Can you work these out from the model? Positions are in its coordinate system, mm. A direction names the side the tool comes from. Give positions to 0.01 mm unless a question says otherwise; leave off trailing zeros. Order: outer loops, then holes, each group sorted by start corner. A loop starts at its lowest first (then second) coordinate and runs counter-clockwise, first axis right, second up. Notation, with made-up numbers: (-19, -1.5) -> (-12, -1.5) arc R29 ccw to (-12, 35.5) -> close; hole circle Ø1 at (-1.75, 15). An arc over 180 degrees is marked (long way). Answer as a JSON object with one key per item and string values.
```python
from build123d import *

# Parameters (mm, degrees)
F0_W      = 37.719
F0_H      = 37.719
F1_DEPTH  = 2.794
F2_W      = 31.75
F2_H      = 31.75
F3_DEPTH  = 10.16
F4_SIZE   = 1.27
F5_W      = 13.843
F5_H      = 31.75
F6_DEPTH  = 7.62
F7_W      = 3.175
F7_H      = 24.6046739221
F7_H_2    = 3.0808845013
F8_DEPTH  = 12.955
F9_W      = 3.1516091073
F9_H      = 27.5891739221
F10_DEPTH = 20.575
F11_DEPTH = 0.762


# Not quite as in the source:
# - a feature names something its author has since deleted; it is built from what else it names


with BuildPart() as f1:
    # F0 (on Front) → F1 (new body)
    with BuildSketch(Plane.XZ):
        Rectangle(F0_W, F0_H)
    extrude(amount=F1_DEPTH)

    # F2 (on face) → F3 (join)
    with BuildSketch(Plane.XZ.offset(2.794)):
        Rectangle(F2_W, F2_H)
    extrude(amount=F3_DEPTH)

    # F4
    f4_edges = [f1.edges().sort_by_distance(p)[0] for p in [
        (-18.8595, -2.794, 0),
        (0, -2.794, -18.8595),
        (18.8595, -2.794, 0),
        (0, -2.794, 18.8595),
    ]]
    chamfer(f4_edges, length=F4_SIZE)

    # F5 (on face) → F6 (join)
    with BuildSketch(Plane.XZ.offset(12.954)):
        with Locations((-8.9535, 0)):
            Rectangle(F5_W, F5_H)
    extrude(amount=F6_DEPTH)

    # F7 (on face) → F8 (cut, through all)
    with BuildSketch(Plane.XZ.offset(12.954)):
        with Locations((2.0955, 3.572663039)):
            Rectangle(F7_W, F7_H)
        with Locations((2.0955, 17.4154422507)):
            Rectangle(F7_W, F7_H_2)
    extrude(amount=-F8_DEPTH, mode=Mode.SUBTRACT)

    # F9 (on face) → F10 (cut, through all)
    with BuildSketch(Plane(origin=(0, 0, 0), x_dir=(-1, 0, 0), z_dir=(0, 1, 0))):
        with Locations((-2.0838045536, 5.064913039)):
            Rectangle(F9_W, F9_H)
    extrude(amount=-F10_DEPTH, mode=Mode.SUBTRACT)

    # F11 (add): a face of the model
    f11_faces = [f1.faces().sort_by_distance(p)[0] for p in [
        (-0.1374824949, 0, -0.3323010646),
    ]]
    extrude(f11_faces, amount=F11_DEPTH)


solid = f1.part
```
1. Will these pins go through, and if not, where does the flat tip stop? pin 1 Ø19.5 at (x, z) = (8, 5.5) entering from -Y; pin 2 Ø5.5 at (x, y) = (-7, -10.5) entering from -Z (3 decimals); pin 3 Ø3.5 at (x, y) = (2.5, -4) entering from +Z.
Worked answers:
{"pin 1": "y = -12.95", "pin 2": "z = -15.875", "pin 3": "z = 17.67"}
2. If we section it at D-D on z = -11: Please give me the cut outline in (x, y) (1 decimal), then the cut area to 3 significant figures.
Worked answers:
{"outline": "(-18.9, -1.5) -> (-17.6, -2.8) -> (-15.9, -2.8) -> (-15.9, -20.6) -> (-2, -20.6) -> (-2, -13) -> (15.9, -13) -> (15.9, -2.8) -> (17.6, -2.8) -> (18.9, -1.5) -> (18.9, 0.8) -> (-18.9, 0.8) -> close", "area": "561 mm²"}
3. Please list where these lines run through material, in increasing order: L1, parallel to X at y = -4.25, z = 5 (3 decimals); L2, parallel to X at y = -17.25, z = -10 (3 decimals); L3, parallel to Y at x = 7.5, z = 8.
Worked answers:
{"L1": "-15.875 to 0.508, 3.683 to 15.875", "L2": "-15.875 to -2.032", "L3": "-12.95 to 0.76"}
4. If we section it at C-C on y = -6.25: Please give me the cut outline in (x, z) (3 decimals).
Worked answers:
{"outline": "(-15.875, -15.875) -> (15.875, -15.875) -> (15.875, 15.875) -> (3.683, 15.875) -> (3.683, -8.73) -> (0.508, -8.73) -> (0.508, 15.875) -> (-15.875, 15.875) -> close"}
5. For faces 1 (the face through (-4, -10, -15.875)), 2 (the face through (9, -12.954, 0)), 3 (the face through (-15.875, -12, 0)), which set-ups out of +Z, -Z, +X, -X, +Y, -Y let a thin tool reach every point of the face, with its end or its side?
Worked answers:
{"face 1": "-Z, +X, -X, -Y", "face 2": "+Z, -Z, +X, -Y", "face 3": "+Z, -Z, -X, -Y"}
6. If we section it at A-A on z = 3.5: Please give me the cut outline in (x, y) (1 decimal).
Worked answers:
{"outline": "(-18.9, -1.5) -> (-17.6, -2.8) -> (-15.9, -2.8) -> (-15.9, -20.6) -> (-2, -20.6) -> (-2, -13) -> (0.5, -13) -> (0.5, 0.8) -> (-18.9, 0.8) -> close; (3.7, -13) -> (15.9, -13) -> (15.9, -2.8) -> (17.6, -2.8) -> (18.9, -1.5) -> (18.9, 0.8) -> (3.7, 0.8) -> close"}
7. If we mould it in two halves opening along X, with no side actions, what happens to faces 4 (the face through (-2.032, -17, 0)), 5 (the face through (3.683, -6, 5)), 6 (the face through (-9.311, -2.168, 18.216))? For each: +X half, -X half, draft (parallel to the pull), parting line (faces both ways), or undercut.
Worked answers:
{"face 4": "+X half", "face 5": "undercut", "face 6": "draft"}
8. If we section it at B-B on x = -3.5: Please give me the cut outline in (y, z) (1 decimal), then the cut area to 3 significant figures.
Worked answers:
{"outline": "(-20.6, -15.9) -> (-2.8, -15.9) -> (-2.8, -17.6) -> (-1.5, -18.9) -> (0.8, -18.9) -> (0.8, 18.9) -> (-1.5, 18.9) -> (-2.8, 17.6) -> (-2.8, 15.9) -> (-20.6, 15.9) -> close", "area": "697 mm²"}
